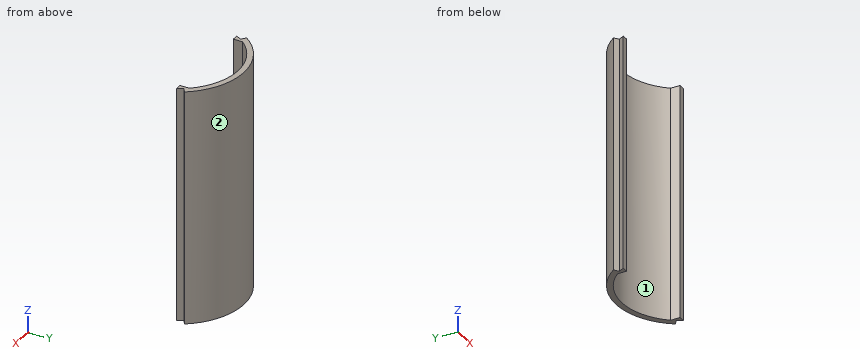
```python
from build123d import *
from build123d.topology import SkipClean

# Parameters (mm, degrees)
SKETCH1_R           = 22.5
SKETCH1_R_2         = 20.5
BOSS_EXTRUDE1_DEPTH = 80
SKETCH2_W           = 45
SKETCH2_H           = 22.5
CUT_EXTRUDE1_DEPTH  = 87.095876789
SKETCH4_W           = 4.401808348
SKETCH4_H           = 1
SKETCH4_W_2         = 1
SKETCH4_H_2         = 3
BOSS_EXTRUDE2_DEPTH = 80
BOSS_EXTRUDE3_START = -80
BOSS_EXTRUDE3_DEPTH = 80
CUT_EXTRUDE2_DEPTH  = 87.095876789


with BuildPart() as part:
    # Sketch1 → Boss-Extrude1 (new body)
    with BuildSketch(Plane.XY):
        Circle(SKETCH1_R)
        Circle(SKETCH1_R_2, mode=Mode.SUBTRACT)
    extrude(amount=BOSS_EXTRUDE1_DEPTH)

    # Sketch2 → Cut-Extrude1 (cut, through all)
    with BuildSketch(Plane.XY.offset(80)):
        with Locations((0, 11.25)):
            Rectangle(SKETCH2_W, SKETCH2_H)
    extrude(amount=-CUT_EXTRUDE1_DEPTH, mode=Mode.SUBTRACT)


with BuildPart() as body_2:
    # Sketch4 → Boss-Extrude2 (new body)
    with BuildSketch(Plane.XY.offset(80)):
        with BuildLine():
            ThreePointArc((22.5, 0), (21.654908627, 6.108594957), (19.183117125, 11.758316945))
            Line((19.183117125, 11.758316945), (19.183117125, 8.758316945))
            Line((19.183117125, 8.758316945), (18.534882905, 8.758316945))
            ThreePointArc((18.534882905, 8.758316945), (20.002688564, 4.488034116), (20.5, 0))
            Line((20.5, 0), (22.5, 0))
        make_face()
        Polygon((16.792616908, 11.758316945), (18.430920997, 12.905469818), (19.183117125, 11.758316945), align=None)
        with BuildLine():
            Line((19.183117125, 8.758316945), (19.183117125, 11.758316945))
            Line((19.183117125, 11.758316945), (16.792616908, 11.758316945))
            ThreePointArc((16.792616908, 11.758316945), (17.439231391, 10.776047906), (18.028456684, 9.758316945))
            ThreePointArc((18.028456684, 9.758316945), (18.288505966, 9.261778962), (18.534882905, 8.758316945))
            Line((18.534882905, 8.758316945), (19.183117125, 8.758316945))
        make_face()
        with BuildLine():
            Line((15.792616908, 9.758316945), (15.792616908, 11.758316945))
            Line((15.792616908, 11.758316945), (14.792616908, 11.758316945))
            Line((14.792616908, 11.758316945), (14.792616908, 8.758316945))
            Line((14.792616908, 8.758316945), (18.534882905, 8.758316945))
            ThreePointArc((18.534882905, 8.758316945), (18.288505966, 9.261778962), (18.028456684, 9.758316945))
            Line((18.028456684, 9.758316945), (15.792616908, 9.758316945))
        make_face()
        with BuildLine():
            Line((-16.702272837, 11.886298081), (-18.340620511, 13.033481472))
            ThreePointArc((-18.340620511, 13.033481472), (-21.43494765, 6.840542322), (-22.5, 0))
            Line((-22.5, 0), (-20.5, 0))
            ThreePointArc((-20.5, 0), (-19.527501033, 6.239126815), (-16.702272837, 11.886298081))
        make_face()
        with Locations((-16.903177011, 9.386298081)):
            Rectangle(SKETCH4_W, SKETCH4_H)
        with Locations((-15.202272837, 10.386298081)):
            Rectangle(SKETCH4_W_2, SKETCH4_H_2)
    extrude(amount=-BOSS_EXTRUDE2_DEPTH)

    # Sketch5 → Boss-Extrude3 (add)
    with SkipClean():  # the faces are left unmerged after this step: merging them gives an invalid solid
        with BuildSketch(Plane.XY.offset(80).offset(BOSS_EXTRUDE3_START)):
            with BuildLine():
                Line((16.792616908, 14.391966981), (16.792616908, 11.758316945))
                Line((16.792616908, 11.758316945), (18.430920997, 12.905469818))
                ThreePointArc((18.430920997, 12.905469818), (0.078328094, 22.49986366), (-18.340620511, 13.033481472))
                Line((-18.340620511, 13.033481472), (-16.702272837, 11.886298081))
                Line((-16.702272837, 11.886298081), (-16.702272837, 13.843152405))
                Line((-16.702272837, 13.843152405), (-15.702272837, 13.843152405))
                Line((-15.702272837, 13.843152405), (-15.702272837, 13.179098139))
                ThreePointArc((-15.702272837, 13.179098139), (0.070554536, 20.499878586), (15.792616908, 13.070702016))
                Line((15.792616908, 13.070702016), (15.792616908, 14.391966981))
                Line((15.792616908, 14.391966981), (16.792616908, 14.391966981))
            make_face()
            with BuildLine():
                Line((15.792616908, 11.758316945), (16.792616908, 11.758316945))
                ThreePointArc((16.792616908, 11.758316945), (16.30582578, 12.424574264), (15.792616908, 13.070702016))
                Line((15.792616908, 13.070702016), (15.792616908, 11.758316945))
            make_face()
            with BuildLine():
                ThreePointArc((15.792616908, 13.070702016), (16.30582578, 12.424574264), (16.792616908, 11.758316945))
                Line((16.792616908, 11.758316945), (16.792616908, 14.391966981))
                Line((16.792616908, 14.391966981), (15.792616908, 14.391966981))
                Line((15.792616908, 14.391966981), (15.792616908, 13.070702016))
            make_face()
            Polygon((17.889582419, 9.858316945), (16.792616908, 11.758316945), (15.792616908, 11.758316945), (15.792616908, 9.858316945), align=None)
            Polygon((-15.702272837, 11.886298081), (-15.702272837, 9.986298081), (-17.799238349, 9.986298081), (-16.702272837, 11.886298081), align=None)
            with BuildLine():
                Line((-15.702272837, 11.886298081), (-15.702272837, 13.179098139))
                ThreePointArc((-15.702272837, 13.179098139), (-16.215161982, 12.542668054), (-16.702272837, 11.886298081))
                Line((-16.702272837, 11.886298081), (-15.702272837, 11.886298081))
            make_face()
            with BuildLine():
                ThreePointArc((-16.702272837, 11.886298081), (-16.215161982, 12.542668054), (-15.702272837, 13.179098139))
                Line((-15.702272837, 13.179098139), (-15.702272837, 13.843152405))
                Line((-15.702272837, 13.843152405), (-16.702272837, 13.843152405))
                Line((-16.702272837, 13.843152405), (-16.702272837, 11.886298081))
            make_face()
        extrude(amount=BOSS_EXTRUDE3_DEPTH)


with BuildPart() as cut_extrude2_tool:
    # Sketch6 → Cut-Extrude2 (new, through all)
    with BuildSketch(Plane.XY.offset(80)):
        with BuildLine():
            Line((-22.5, 0), (-20.5, 0))
            ThreePointArc((-20.5, 0), (-19.98704884, 4.557178804), (-18.473865497, 8.886298081))
            Line((-18.473865497, 8.886298081), (-19.42662195, 8.886298081))
            Line((-19.42662195, 8.886298081), (-19.42662195, 9.886298081))
            Line((-19.42662195, 9.886298081), (-17.958594328, 9.886298081))
            ThreePointArc((-17.958594328, 9.886298081), (-17.359260588, 10.904406074), (-16.702272837, 11.886298081))
            Line((-16.702272837, 11.886298081), (-18.33176287, 13.045936918))
            ThreePointArc((-18.33176287, 13.045936918), (-21.432623085, 6.847822114), (-22.5, 0))
        make_face()
        with BuildLine():
            Line((22.5, 0), (20.5, 0))
            ThreePointArc((20.5, 0), (0, -20.5), (-20.5, 0))
            Line((-20.5, 0), (-22.5, 0))
            ThreePointArc((-22.5, 0), (0, -22.5), (22.5, 0))
        make_face()
        with BuildLine():
            Line((-19.42662195, 8.886298081), (-18.473865497, 8.886298081))
            ThreePointArc((-18.473865497, 8.886298081), (-18.223090634, 9.389833213), (-17.958594328, 9.886298081))
            Line((-17.958594328, 9.886298081), (-19.42662195, 9.886298081))
            Line((-19.42662195, 9.886298081), (-19.42662195, 8.886298081))
        make_face()
        with BuildLine():
            ThreePointArc((-17.958594328, 9.886298081), (-18.223090634, 9.389833213), (-18.473865497, 8.886298081))
            Line((-18.473865497, 8.886298081), (-15.702272837, 8.886298081))
            Line((-15.702272837, 8.886298081), (-15.702272837, 9.886298081))
            Line((-15.702272837, 9.886298081), (-17.958594328, 9.886298081))
        make_face()
        Polygon((-15.702272837, 9.886298081), (-15.702272837, 8.886298081), (-14.702272837, 8.886298081), (-14.702272837, 11.886298081), (-15.702272837, 11.886298081), (-15.702272837, 9.986298081), align=None)
        Polygon((15.792616908, 11.758316945), (14.792616908, 11.758316945), (14.792616908, 8.758316945), (15.792616908, 8.758316945), (15.792616908, 9.758316945), (15.792616908, 9.858316945), align=None)
        with BuildLine():
            Line((15.792616908, 9.758316945), (15.792616908, 8.758316945))
            Line((15.792616908, 8.758316945), (18.534882905, 8.758316945))
            ThreePointArc((18.534882905, 8.758316945), (18.288505966, 9.261778962), (18.028456684, 9.758316945))
            Line((18.028456684, 9.758316945), (15.792616908, 9.758316945))
        make_face()
        with BuildLine():
            ThreePointArc((18.028456684, 9.758316945), (18.288505966, 9.261778962), (18.534882905, 8.758316945))
            Line((18.534882905, 8.758316945), (19.161355292, 8.758316945))
            Line((19.161355292, 8.758316945), (19.161355292, 9.758316945))
            Line((19.161355292, 9.758316945), (18.028456684, 9.758316945))
        make_face()
        with BuildLine():
            Line((19.161355292, 8.758316945), (18.534882905, 8.758316945))
            ThreePointArc((18.534882905, 8.758316945), (20.002688564, 4.488034116), (20.5, 0))
            Line((20.5, 0), (22.5, 0))
            ThreePointArc((22.5, 0), (21.654908627, 6.108594957), (19.183117125, 11.758316945))
            Line((19.183117125, 11.758316945), (18.430920997, 12.905469818))
            Line((18.430920997, 12.905469818), (16.792616908, 11.758316945))
            ThreePointArc((16.792616908, 11.758316945), (17.439231391, 10.776047906), (18.028456684, 9.758316945))
            Line((18.028456684, 9.758316945), (19.161355292, 9.758316945))
            Line((19.161355292, 9.758316945), (19.161355292, 8.758316945))
        make_face()
    extrude(amount=-CUT_EXTRUDE2_DEPTH)


with BuildPart() as part_1:
    add(part.part)

    # Cut-Extrude2: cut by cut_extrude2_tool
    add(cut_extrude2_tool.part, mode=Mode.SUBTRACT)


with BuildPart() as body_2_1:
    add(body_2.part)

    # Cut-Extrude2: cut by cut_extrude2_tool
    add(cut_extrude2_tool.part, mode=Mode.SUBTRACT)


solid = body_2_1.part
```
Design review of the part built by this model. Coordinates are the model's own, in mm. Face numbers are marked on the shaded views. Give positions to 0.01 mm unless a question says otherwise; leave off trailing zeros. Order: outer loops, then holes, each group sorted by start corner. A loop starts at its lowest first (then second) coordinate and runs counter-clockwise, first axis right, second up. Notation, with made-up numbers: (-2.75, 2) - (51.25, 2) arc R18 ccw to (51.25, 37) - close; hole circle Ø6 at (12.25, -31). An arc over 180 degrees is marked (long way). Use a Markdown table: item, result. Add a question column.
(1) Wall thickness on probe 1 along X at (y, z) = (13.25, 58); probe 2 along X at (y, z) = (15.75, 19); probe 3 along Y at (x, z) = (-3.5, 57): over which ranges is each line inside the solid? List them lowest first. Write a range as [from, to].
(2) Add section D-D on x = 4. Give the boundary of the cut face in (y, z).
(3) Add section C-C on y = 10.75. Give the boundary of the cut face in (x, z).
(4) Clearance check with flat-ended pins moving along their axes: P1, Ø1.6, axis at y = 11.5, z = 30.5, coming from the -X side; P2, Ø2.5, axis at x = -16.5, z = 45.5, coming from the -Y side; P3, Ø12, axis at x = 10, z = 17.5, coming from the +Y side. State where each tip first meets the part, or that it passes through.
(5) Add section B-B on y = 17. Give the boundary of the cut face in (x, z), then the cut area to 3 significant figures.
(6) Mouldability with a two-part tool opening along X and no side actions: class the marked faces 1 and 2 as +X half, -X half, draft (parallel to the pull), parting line (faces both ways), or undercut.
(7) Add section A-A on z = 42. Give the boundary of the cut face in (x, y).
Report:
| question | item | result |
|---|---|---|
| 1 | probe 1 | x = [-18.18, -15.64], [15.64, 18.18] |
| 1 | probe 2 | x = [-16.07, -13.12], [13.12, 16.07] |
| 1 | probe 3 | y = [20.2, 22.23] |
| 2 | outline | (20.11, 0) - (22.14, 0) - (22.14, 80) - (20.11, 80) - close |
| 3 | outline | (-17.36, 0) - (-15.7, 0) - (-15.7, 80) - (-17.36, 80) - close; (15.79, 0) - (17.37, 0) - (17.37, 80) - (15.79, 80) - close |
| 4 | P1 | stops at x = -17.39 |
| 4 | P2 | stops at y = 9.99 |
| 4 | P3 | stops at y = 22.14 |
| 5 | outline | (-14.74, 0) - (-11.46, 0) - (-11.46, 80) - (-14.74, 80) - close; (11.46, 0) - (14.74, 0) - (14.74, 80) - (11.46, 80) - close |
| 5 | area | 525 mm² |
| 6 | face 1 | undercut |
| 6 | face 2 | parting line |
| 7 | outline | (-18.33, 13.05) - (-16.7, 11.89) - (-17.8, 9.99) - (-15.7, 9.99) - (-15.7, 13.18) arc R20.5 cw to (15.79, 13.07) - (15.79, 9.86) - (17.89, 9.86) - (16.79, 11.76) - (18.43, 12.91) arc R22.5 ccw to start |
